Check sheet for the modelled part. Datum: model origin and axes. Units: mm. Round coordinates to 2 decimals unless told otherwise and drop trailing zeros. Write each loop counter-clockwise with the first axis right and the second up, starting at its lowest first coordinate (ties: lowest second). Pieces come first, ordered by that corner, then holes.
Item 1: Cross-section at D-D on y = 25. Enter the section's corners in (x, z), plus the area to 3 significant figures.
Item 2: Cross-section at C-C on z = 7.5. Enter the section's corners in (x, y), plus the area to 3 significant figures.
Item 3: Cross-section at B-B on z = 25. Enter the section's corners in (x, y).
Item 4: Go/stop test with flat-tipped pins: pin 1 Ø1 at (x, y) = (1, 31.5) entering from +Z; pin 2 Ø2 at (y, z) = (6, 8.5) entering from -X; pin 3 Ø0.6 at (x, z) = (0.5, 25) entering from +Y. Record where each tip stops, or that it passes through.
Item 5: Material ranges on line 1 (Y direction, x = 0.9, z = 7.5); line 2 (Z direction, x = 0.9, y = 10); line 3 (Z direction, x = 1.05, y = 25), recorded low to high.
Item 6: Cross-section at A-A on y = 10. Enter the section's corners in (x, z).
Autodesk Inventor part; units mm, degrees
ref_plane "YZ Plane" through (0, 0, 0) normal (1, 0, 0) x (0, 1, 0)
ref_plane "XZ Plane" through (0, 0, 0) normal (0, 1, 0) x (-1, 0, 0)
ref_plane "XY Plane" through (0, 0, 0) normal (0, 0, 1) x (1, 0, 0)
sketch "スケッチ1" plane through (0, 0, 0) normal (1, 0, 0) x (0, 1, 0)
  line L0 (0, 0) -> (50, 0)
  line L1 (50, 0) -> (50, 15)
  line L2 (50, 15) -> (0, 15)
  line L3 (0, 15) -> (0, 0)
  line L4 (0, 0) -> (20, 0)
  line L5 (20, 0) -> (20, 30)
  line L6 (20, 30) -> (0, 30)
  line L7 (0, 30) -> (0, 0)
  point P0 (0, 15)
  point P1 (20, 15)
  point P2 (20, 0)
  point P3 (20, 0)
  dimension "d0" = 15
  dimension "d1" = 20
  dimension "d2" = 30
  dimension "d3" = 30
extrude "押し出し1" add sketch "スケッチ1" along normal blind 2
sketch "スケッチ2" plane through (2, 0, 0) normal (1, 0, 0) x (0, 0, -1)
  line L0 (-30, 20) -> (-30, 0)
  line L1 (-30, 10) -> (0, 10) construction
  line L2 (0, 0) -> (0, 50)
  line L3 (0, 50) -> (-15, 50)
  line L4 (-7.5, 50) -> (-7.5, 0) construction
  line L5 (-30, 0) -> (0, 0)
  point P0 (-25, 10)
  point P1 (-5, 10)
  point P2 (-7.5, 25)
  point P3 (-7.5, 45)
  dimension "d6" = 20
  dimension "d7" = 5
  dimension "d8" = 20
  dimension "d9" = 5
hole "穴1" at (2, 10, 25) at (2, 10, 5) at (2, 25, 7.5) at (2, 45, 7.5) direction (-1, 0, 0) diameter 3.2 end through all
properties part number "FrameJointL2015" material "アルミニウム 6061"
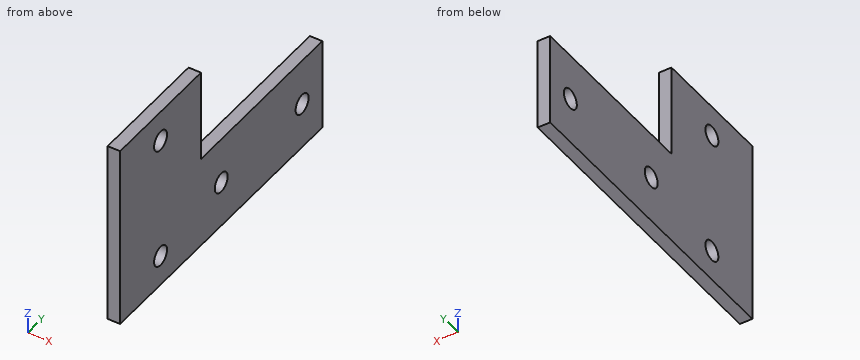
Response values:
1. outline: (0, 0) - (2, 0) - (2, 5.9) - (0, 5.9) - close; (0, 9.1) - (2, 9.1) - (2, 15) - (0, 15) - close
1. area: 23.6 mm2
2. outline: (0, 0) - (2, 0) - (2, 23.4) - (0, 23.4) - close; (0, 26.6) - (2, 26.6) - (2, 43.4) - (0, 43.4) - close; (0, 46.6) - (2, 46.6) - (2, 50) - (0, 50) - close
2. area: 87.2 mm2
3. outline: (0, 0) - (2, 0) - (2, 8.4) - (0, 8.4) - close; (0, 11.6) - (2, 11.6) - (2, 20) - (0, 20) - close
4. pin 1: stops at z = 15
4. pin 2: stops at x = 0
4. pin 3: stops at y = 20
5. line 1: y = 0 to 23.4, 26.6 to 43.4, 46.6 to 50
5. line 2: z = 0 to 3.4, 6.6 to 23.4, 26.6 to 30
5. line 3: z = 0 to 5.9, 9.1 to 15
6. outline: (0, 0) - (2, 0) - (2, 3.4) - (0, 3.4) - close; (0, 6.6) - (2, 6.6) - (2, 23.4) - (0, 23.4) - close; (0, 26.6) - (2, 26.6) - (2, 30) - (0, 30) - close
